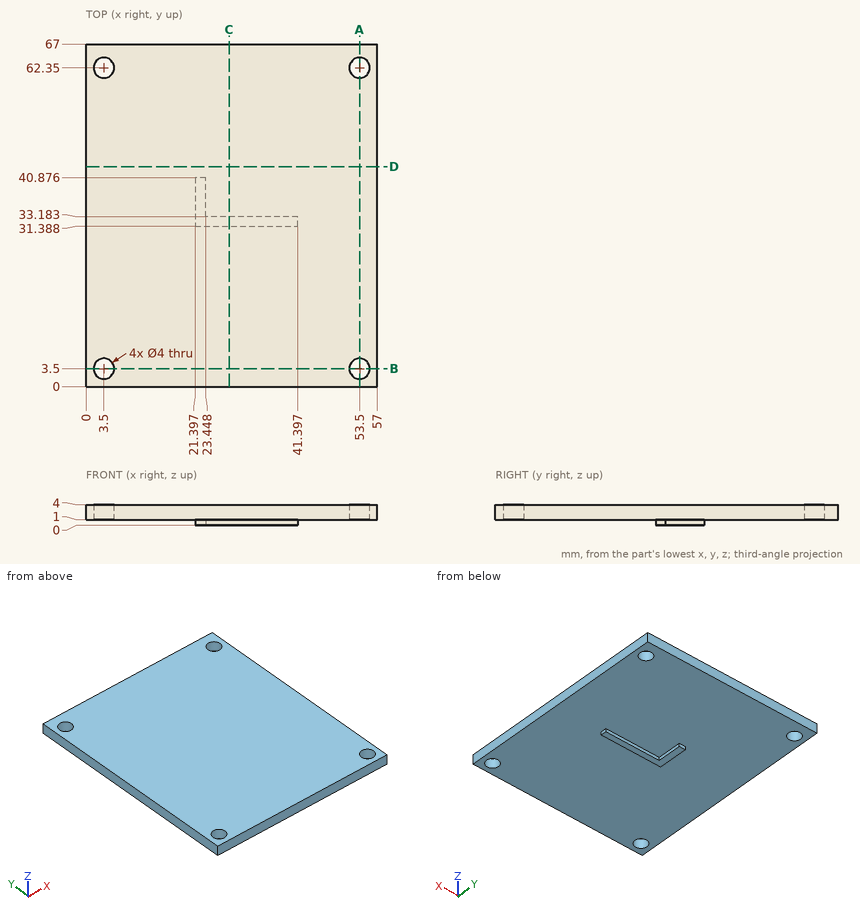
Source: three-view drawing plus pictorial views. Frame: mm from the lowest corner of the part. Give positions to 0.01 mm unless a question says otherwise; leave off trailing zeros. Write each loop counter-clockwise with the first axis right and the second up, starting at its lowest first coordinate (ties: lowest second). Pieces come first, ordered by that corner, then holes.
(1) Ray query, line 1 (Y direction, x = 3.5, z = 1.9); line 2 (Z direction, x = 10.5, y = 58). Return the intervals inside material, ascending.
(2) Cut plane B-B, the plane y = 3.5. Return loops of the section in (x, z).
(3) Cut plane C-C, the plane x = 28. Return loops of the section in (y, z).
(4) Cut plane D-D, the plane y = 43. Return loops of the section in (x, z), then the cut area to 3 significant figures.
(5) Cut plane A-A, the plane x = 53.5. Return loops of the section in (y, z), then the cut area to 3 significant figures.
(6) First-contact query: P1, Ø8, axis at x = 25.5, y = 19.5, coming from the -Z side; P2, Ø0.8, axis at y = 35.5, z = 0.5, coming from the +X side; P3, Ø0.5, axis at x = 22.5, z = 0.5, coming from the +Y side; P4, Ø3.5, axis at x = 3.5, y = 62.35, coming from the -Z side. Flat tips, straight axial feed; report the tip coordinate or a pass-through.
Values follow:
1. line 1: y = 0 to 1.5, 5.5 to 60.35, 64.35 to 67
1. line 2: z = 1 to 4
2. outline: (0, 1) - (1.5, 1) - (1.5, 4) - (0, 4) - close; (5.5, 1) - (51.5, 1) - (51.5, 4) - (5.5, 4) - close; (55.5, 1) - (57, 1) - (57, 4) - (55.5, 4) - close
3. outline: (0, 1) - (31.39, 1) - (31.39, 0) - (33.18, 0) - (33.18, 1) - (67, 1) - (67, 4) - (0, 4) - close
4. outline: (0, 1) - (57, 1) - (57, 4) - (0, 4) - close
4. area: 171 mm2
5. outline: (0, 1) - (1.5, 1) - (1.5, 4) - (0, 4) - close; (5.5, 1) - (60.35, 1) - (60.35, 4) - (5.5, 4) - close; (64.35, 1) - (67, 1) - (67, 4) - (64.35, 4) - close
5. area: 177 mm2
6. P1: stops at z = 1
6. P2: stops at x = 23.45
6. P3: stops at y = 40.88
6. P4: passes through
